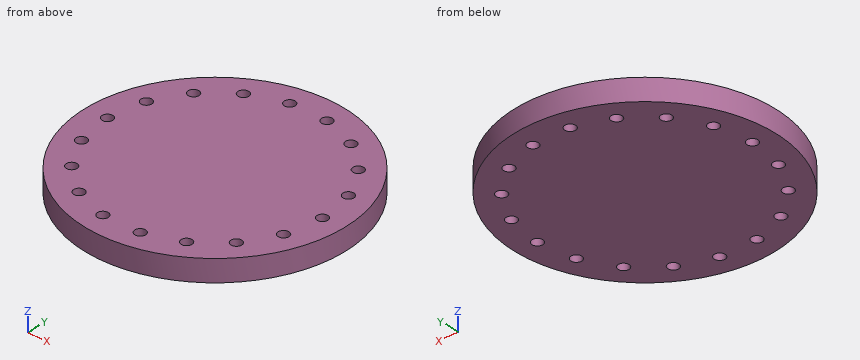
from build123d import *

# Parameters (mm, degrees)
SKETCH1_R           = 76.2
SKETCH1_R_2         = 3.175
BOSS_EXTRUDE1_DEPTH = 12.7


with BuildPart() as part:
    # Sketch1 → Boss-Extrude1 (new body)
    with BuildSketch(Plane.XY):
        Circle(SKETCH1_R)
        with Locations((-63.5, 0)):
            Circle(SKETCH1_R_2, mode=Mode.SUBTRACT)
        with Locations((-59.67048142, 21.718279101)):
            Circle(SKETCH1_R_2, mode=Mode.SUBTRACT)
        with Locations((-48.643822138, 40.817013215)):
            Circle(SKETCH1_R_2, mode=Mode.SUBTRACT)
        with Locations((-31.75, 54.99261314)):
            Circle(SKETCH1_R_2, mode=Mode.SUBTRACT)
        with Locations((-11.026659282, 62.535292316)):
            Circle(SKETCH1_R_2, mode=Mode.SUBTRACT)
        with Locations((11.026659282, 62.535292316)):
            Circle(SKETCH1_R_2, mode=Mode.SUBTRACT)
        with Locations((31.75, 54.99261314)):
            Circle(SKETCH1_R_2, mode=Mode.SUBTRACT)
        with Locations((48.643822138, 40.817013215)):
            Circle(SKETCH1_R_2, mode=Mode.SUBTRACT)
        with Locations((59.67048142, 21.718279101)):
            Circle(SKETCH1_R_2, mode=Mode.SUBTRACT)
        with Locations((63.5, 0)):
            Circle(SKETCH1_R_2, mode=Mode.SUBTRACT)
        with Locations((59.67048142, -21.718279101)):
            Circle(SKETCH1_R_2, mode=Mode.SUBTRACT)
        with Locations((48.643822138, -40.817013215)):
            Circle(SKETCH1_R_2, mode=Mode.SUBTRACT)
        with Locations((31.75, -54.99261314)):
            Circle(SKETCH1_R_2, mode=Mode.SUBTRACT)
        with Locations((11.026659282, -62.535292316)):
            Circle(SKETCH1_R_2, mode=Mode.SUBTRACT)
        with Locations((-11.026659282, -62.535292316)):
            Circle(SKETCH1_R_2, mode=Mode.SUBTRACT)
        with Locations((-31.75, -54.99261314)):
            Circle(SKETCH1_R_2, mode=Mode.SUBTRACT)
        with Locations((-48.643822138, -40.817013215)):
            Circle(SKETCH1_R_2, mode=Mode.SUBTRACT)
        with Locations((-59.67048142, -21.718279101)):
            Circle(SKETCH1_R_2, mode=Mode.SUBTRACT)
    extrude(amount=BOSS_EXTRUDE1_DEPTH)


solid = part.part
Source: CAD feature listing. Evaluate the final solid. Frame: model axes, mm. Coordinates: 2 decimals unless noted, no trailing zeros. Order: outer loops, then holes, each group sorted by start corner. A loop starts at its lowest first (then second) coordinate and runs counter-clockwise, first axis right, second up. Notation, with made-up numbers: M 48,73.25 L 84,73.25 A25 cw 84,109.25 Z; hole C 29.5,83.5 d1. An arc over 180 degrees is marked long. Write each question's results on one line, items separated by ' | '. Start each with the question number.
Item 1: First-contact query: pin 1 Ø6 at (y, z) = (-40, 2.5) entering from +X; pin 2 Ø1 at (x, z) = (-57, 2.5) entering from -Y; pin 3 Ø3 at (x, z) = (-32, 3) entering from +Y. Flat tips, straight axial feed; report the tip coordinate or a pass-through.
Item 2: Cut plane A-A (y = 0). Return loops of the section in (x, z) (3 decimals).
Item 3: Cut plane D-D (x = -26.5). Return loops of the section in (y, z).
Item 4: Cut plane C-C (z = 7). Count the separate pieces of the cut face and the enclosed holes in it, and give its area (3 significant figures).
Item 5: Line query: probe 1 along X at (y, z) = (19.5, 4); probe 2 along Y at (x, z) = (31.75, 8.5); probe 3 along Y at (x, z) = (-31, 11.75). Output: solid intervals per line, ascending.
Item 6: Cut plane B-B (x = 31). Return loops of the section in (y, z), and give its area (3 significant figures).
Checked values:
1) pin 1: stops at x = 66.61 | pin 2: stops at y = -51.13 | pin 3: stops at y = 69.83
2) outline: M -76.2,0 L -66.675,0 L -66.675,12.7 L -76.2,12.7 Z; M -60.325,0 L 60.325,0 L 60.325,12.7 L -60.325,12.7 Z; M 66.675,0 L 76.2,0 L 76.2,12.7 L 66.675,12.7 Z
3) outline: M -71.44,0 L 71.44,0 L 71.44,12.7 L -71.44,12.7 Z
4) separate pieces: 1 | enclosed holes: 18 | area: 17,700 mm2
5) probe 1: x = -73.66 to -61.94, -57.4 to 57.4, 61.94 to 73.66 | probe 2: y = -69.27 to -58.17, -51.82 to 51.82, 58.17 to 69.27 | probe 3: y = -69.61 to -58.08, -51.91 to 51.91, 58.08 to 69.61
6) outline: M -69.61,0 L -58.08,0 L -58.08,12.7 L -69.61,12.7 Z; M -51.91,0 L 51.91,0 L 51.91,12.7 L -51.91,12.7 Z; M 58.08,0 L 69.61,0 L 69.61,12.7 L 58.08,12.7 Z | area: 1,610 mm2
